```python
from build123d import *

# Parameters (mm, degrees)
SCHIZZO1_W                        = 60
SCHIZZO1_H                        = 7.2
SCHIZZO1_W_2                      = 19.125
SCHIZZO1_H_2                      = 5
ESTRUSIONE_ESTRUSIONE1_DEPTH      = 40
SCHIZZO2_W                        = 11.375
SCHIZZO2_H                        = 5
SCHIZZO2_W_2                      = 2.075
SCHIZZO2_H_2                      = 1.1
SCHIZZO2_W_3                      = 2.05
TAGLIO_ESTRUSIONE1_DEPTH          = 61
SMUSSO1_SIZE                      = 0.75
SCHIZZO3_W                        = 7.25
SCHIZZO3_H                        = 5
TAGLIO_ESTRUSIONE2_DEPTH          = 64
SCHIZZO4_W                        = 38.5
SCHIZZO4_H                        = 1.1
ESTRUSIONE_ESTRUSIONE3_DEPTH      = 60
SCHIZZO7_W                        = 30
SCHIZZO7_H                        = 1.1
ESTRUSIONE_ESTRUSIONE4_DEPTH      = 50
ESTRUSIONE_ESTRUSIONE5_DEPTH      = 5
SCHIZZO9_W                        = 19.125
SCHIZZO9_H                        = 1.1
ESTRUSIONE_ESTRUSIONE6_DEPTH      = 5
ESTRUSIONE_ESTRUSIONE6_DEPTH_BACK = 35
SCHIZZO10_W                       = 19.125
SCHIZZO10_H                       = 3.9
TAGLIO_ESTRUSIONE3_DEPTH          = 41
SCHIZZO11_W                       = 19.125
SCHIZZO11_H                       = 7.8
ESTRUSIONE_ESTRUSIONE7_DEPTH      = 40
SCHIZZO12_W                       = 30
SCHIZZO12_H                       = 10
TAGLIO_ESTRUSIONE4_DEPTH          = 64


with BuildPart() as part:
    # Schizzo1 → Estrusione-Estrusione1 (new body)
    with BuildSketch(Plane(origin=(0, 0, 0), x_dir=(0, 0, -1), z_dir=(1, 0, 0))):
        with Locations((30, 3.6)):
            Rectangle(SCHIZZO1_W, SCHIZZO1_H)
        with Locations((43.1875, 3.6)):
            Rectangle(SCHIZZO1_W_2, SCHIZZO1_H_2, mode=Mode.SUBTRACT)
        with Locations((16.8125, 3.6)):
            Rectangle(SCHIZZO1_W_2, SCHIZZO1_H_2, mode=Mode.SUBTRACT)
    extrude(amount=ESTRUSIONE_ESTRUSIONE1_DEPTH)

    # Schizzo2 → Taglio-Estrusione1 (cut, through all)
    with BuildSketch(Plane.XY):
        with Locations((10.6875, 2.5)):
            Rectangle(SCHIZZO2_W, SCHIZZO2_H)
        with Locations((29.3125, 2.5)):
            Rectangle(SCHIZZO2_W, SCHIZZO2_H)
        with Locations((15.3375, 6.65)):
            Rectangle(SCHIZZO2_W_2, SCHIZZO2_H_2)
        with Locations((8.275, 6.65)):
            Rectangle(SCHIZZO2_W_3, SCHIZZO2_H_2)
        with Locations((24.6625, 6.65)):
            Rectangle(SCHIZZO2_W_2, SCHIZZO2_H_2)
        with Locations((31.725, 6.65)):
            Rectangle(SCHIZZO2_W_3, SCHIZZO2_H_2)
    extrude(amount=-TAGLIO_ESTRUSIONE1_DEPTH, mode=Mode.SUBTRACT)

    # Smusso1
    smusso1_edges = [part.edges().sort_by_distance(p)[0] for p in [
        (40, 3.6, 0),
        (0, 3.6, 0),
        (0, 3.6, -60),
        (40, 3.6, -60),
    ]]
    chamfer(smusso1_edges, length=SMUSSO1_SIZE)

    # Schizzo3 → Taglio-Estrusione2 (cut)
    with BuildSketch(Plane.XY):
        with Locations((20, 2.5)):
            Rectangle(SCHIZZO3_W, SCHIZZO3_H)
    extrude(amount=-TAGLIO_ESTRUSIONE2_DEPTH, mode=Mode.SUBTRACT)

    # Schizzo4 → Estrusione-Estrusione3 (add)
    with BuildSketch(Plane.XY):
        with Locations((20, 6.65)):
            Rectangle(SCHIZZO4_W, SCHIZZO4_H)
    extrude(amount=-ESTRUSIONE_ESTRUSIONE3_DEPTH)

    # Schizzo7 → Estrusione-Estrusione4 (add)
    with BuildSketch(Plane.XY.offset(-52.75)):
        with Locations((20, 5.55)):
            Rectangle(SCHIZZO7_W, SCHIZZO7_H)
    extrude(amount=ESTRUSIONE_ESTRUSIONE4_DEPTH)

    # Schizzo8 → Estrusione-Estrusione5 (add)
    with BuildSketch(Plane.XZ):
        Polygon((5, 0), (0.75, 0), (0, -0.75), (0, -59.25), (0.75, -60), (5, -60), align=None)
        Polygon((35, 0), (35, -60), (39.25, -60), (40, -59.25), (40, -0.75), (39.25, 0), align=None)
    extrude(amount=ESTRUSIONE_ESTRUSIONE5_DEPTH)

    # Schizzo9 → Estrusione-Estrusione6 (add, two sides)
    with BuildSketch(Plane(origin=(35, 0, 0), x_dir=(0, 0, -1), z_dir=(1, 0, 0))) as estrusione_estrusione6_sk:
        with Locations((16.8125, 5.55)):
            Rectangle(SCHIZZO9_W, SCHIZZO9_H)
        with Locations((43.1875, 5.55)):
            Rectangle(SCHIZZO9_W, SCHIZZO9_H)
    extrude(amount=ESTRUSIONE_ESTRUSIONE6_DEPTH)
    extrude(estrusione_estrusione6_sk.sketch, amount=-ESTRUSIONE_ESTRUSIONE6_DEPTH_BACK)

    # Schizzo10 → Taglio-Estrusione3 (cut, through all)
    with BuildSketch(Plane.ZY):
        with Locations((-43.1875, -0.85)):
            Rectangle(SCHIZZO10_W, SCHIZZO10_H)
        with Locations((-16.8125, -0.85)):
            Rectangle(SCHIZZO10_W, SCHIZZO10_H)
    extrude(amount=-TAGLIO_ESTRUSIONE3_DEPTH, mode=Mode.SUBTRACT)

    # Schizzo11 → Estrusione-Estrusione7 (add)
    with BuildSketch(Plane.ZY):
        with Locations((-43.1875, 1.1)):
            Rectangle(SCHIZZO11_W, SCHIZZO11_H)
        with Locations((-16.8125, 1.1)):
            Rectangle(SCHIZZO11_W, SCHIZZO11_H)
    extrude(amount=-ESTRUSIONE_ESTRUSIONE7_DEPTH)

    # Schizzo12 → Taglio-Estrusione4 (cut)
    with BuildSketch(Plane(origin=(0, 0, -60), x_dir=(-1, 0, 0), z_dir=(0, 0, -1))):
        with Locations((-20, 0)):
            Rectangle(SCHIZZO12_W, SCHIZZO12_H)
    extrude(amount=-TAGLIO_ESTRUSIONE4_DEPTH, mode=Mode.SUBTRACT)


solid = part.part
```
Read the model definition and answer for the solid it produces. Units are mm, in the model's axes. A direction names the side the tool comes from. Round coordinates to 2 decimals unless told otherwise and drop trailing zeros. Write each loop counter-clockwise with the first axis right and the second up, starting at its lowest first coordinate (ties: lowest second). Pieces come first, ordered by that corner, then holes. Notation, with made-up numbers: (6.25, 43.25) -> (63.25, 43.25) arc R16 ccw to (63.25, 56.25) -> close; hole circle Ø10 at (77, -8). An arc over 180 degrees is marked (long way). Answer in a Markdown table with one row per item. Add a question column.
1) Consider line 1 (X direction, y = -3.25, z = -5); line 2 (Y direction, x = 25, z = -11). Determine where each line is inside the solid, lowest interval first.
2) Find section A-A, the plane y = 0.75. Determine the outline of the cut face in (x, z), and give its area (3 significant figures).
3) Determine the mould class of faces 3 (the face through (20, 5, -30)), 4 (the face through (0, 1, -30)), 5 (the face through (20, 7.2, -30)) for opening direction X: pulls with the +X half, pulls with the -X half, needs draft (parallel to the pull), parting line crosses it, or undercut.
4) Find section C-C, the plane x = 25. Determine the outline of the cut face in (y, z).
5) Find section B-B, the plane z = -5. Determine the outline of the cut face in (x, y), and give its area (3 significant figures).
6) Which of the six approach directions +Z, -Z, +X, -X, +Y, -Y give full straight-line access (tool end or side, diameter ignored) to faces 1 (the face through (35, 0, -30)), 2 (the face through (20.3, 5.3, 0))?
7) Given P1, Ø24, axis at x = 20.5, z = -17, coming from the -Y side, flat-ended and moving along its own axis, determine where the tip first touches the part or whether it passes through.
Findings below:
| question | item | result |
|---|---|---|
| 1 | line 1 | 0 to 5, 35 to 40 |
| 1 | line 2 | 5 to 7.2 |
| 2 | outline | (0, -59.25) -> (0.75, -60) -> (5, -60) -> (5, 0) -> (0.75, 0) -> (0, -0.75) -> close; (35, -60) -> (39.25, -60) -> (40, -59.25) -> (40, -0.75) -> (39.25, 0) -> (35, 0) -> close |
| 2 | area | 599 mm² |
| 3 | face 3 | undercut |
| 3 | face 4 | pulls with the -X half |
| 3 | face 5 | needs draft |
| 4 | outline | (5, -60) -> (7.2, -60) -> (7.2, 0) -> (5, 0) -> close |
| 5 | outline | (0, -5) -> (5, -5) -> (5, 5) -> (35, 5) -> (35, -5) -> (40, -5) -> (40, 7.2) -> (0, 7.2) -> close |
| 5 | area | 188 mm² |
| 6 | face 1 | +Z, -Z, -Y |
| 6 | face 2 | +Z, +X, -X, +Y, -Y |
| 7 | P1 | y = 5 |
